Check sheet for the modelled part. Datum: model origin and axes. Units: mm. Face numbers are marked on the shaded views. A direction names the side the tool comes from. Give positions to 0.01 mm unless a question says otherwise; leave off trailing zeros. Loops run counter-clockwise (first coordinate to the right, second up) from the corner with the lowest first, then second, coordinate; pieces in that order, holes last. Notation, with made-up numbers: (-18.75, -13) - (6.25, -13) arc R17 cw to (6.25, 17) - close; hole circle Ø9 at (55, 9.5). An arc over 180 degrees is marked (long way). Use CSV: the item, a comma, the result in double quotes.
from build123d import *

# Parameters (mm, degrees)
F0_R     = 12.75
F1_DEPTH = 2
F2_SIZE  = 1.99999
F3_R     = 4
F4_DEPTH = 3.5


# Not quite as in the source:
# - a fillet or chamfer is up to 0.001 mm smaller than in the source, because OpenCascade refuses the exact size


with BuildPart() as f1:
    # F0 (on Top) → F1 (new body)
    with BuildSketch(Plane.XY):
        Circle(F0_R)
    extrude(amount=F1_DEPTH)

    # F2 (size 2 in the source; OpenCascade refuses exactly that, so slightly less here)
    f2_edges = [f1.edges().sort_by_distance(p)[0] for p in [
        (-12.75, 0, 0),
    ]]
    chamfer(f2_edges, length=F2_SIZE)

    # F3 (on face) → F4 (join)
    with BuildSketch(Plane(origin=(0, 0, 0), x_dir=(1, 0, 0), z_dir=(0, 0, -1))):
        Circle(F3_R)
    extrude(amount=F4_DEPTH)


solid = f1.part
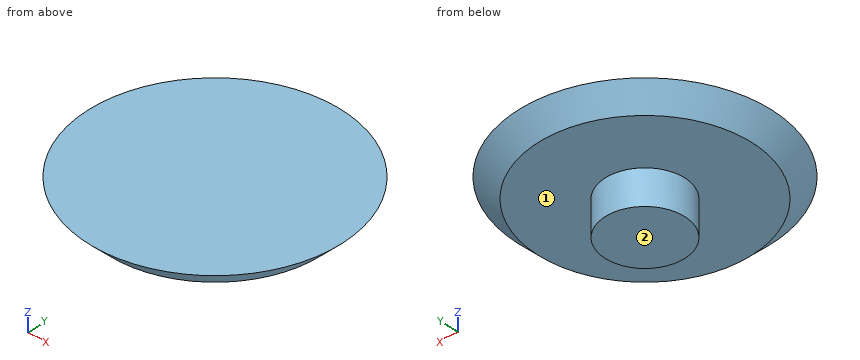
1. Go/stop test with a flat-tipped pin: pin 1 Ø2 at (x, z) = (-5, 1) entering from -Y. Record where the tip stops, or that it passes through.
Completed:
pin 1,"stops at y = -11.8"
2. Set-up check for the marked faces 1 and 2: record each of +Z, -Z, +X, -X, +Y, -Y from which the full face is reachable in a straight line by a thin tool's end or side.
Completed:
face 1,"-Z"
face 2,"-Z, +X, -X, +Y, -Y"
3. Sectioned sample at D-D, the plane z = -1.5. Record the boundary of the cut face in (x, y), and give its area (3 significant figures).
Completed:
outline,"circle Ø8 at (0, 0)"
area,"50.3 mm²"
4. Scan lines: line 1 along Z through (x, y) = (7.25, 1); line 2 along Y through (x, z) = (-5.75, 0.8); line 3 along X through (y, z) = (1.75, -2.25). Record each from-to range of solid material in increasing order.
Completed:
line 1,"z = 0 to 2"
line 2,"y = -10.02 to 10.02"
line 3,"x = -3.6 to 3.6"
5. Sectioned sample at C-C, the plane z = 1.2. Record the boundary of the cut face in (x, y), and give its area (3 significant figures).
Completed:
outline,"circle Ø23.9 at (0, 0)"
area,"449 mm²"
